Read the model definition and answer for the solid it produces. Units are mm, in the model's axes. Give positions to 0.01 mm unless a question says otherwise; leave off trailing zeros. Write each loop counter-clockwise with the first axis right and the second up, starting at its lowest first coordinate (ties: lowest second). Pieces come first, ordered by that corner, then holes. Notation, with made-up numbers: (52, 12) -> (69, 12) arc R30 ccw to (69, 50) -> close; hole circle Ø7 at (0.25, 11.25). An arc over 180 degrees is marked (long way). Use a Markdown table: item, result.
from build123d import *

# Parameters (mm, degrees)
F0_R     = 10.25
F0_R_2   = 11.173899
F1_DEPTH = 40


with BuildPart() as f1:
    # F0 (on Top) → F1 (new body)
    with BuildSketch(Plane.XY):
        with BuildLine():
            Line((-240, -166), (240, -166))
            ThreePointArc((240, -166), (247.071068, -163.071068), (250, -156))
            Line((250, -156), (250, 156))
            ThreePointArc((250, 156), (247.071068, 163.071068), (240, 166))
            Line((240, 166), (-240, 166))
            ThreePointArc((-240, 166), (-247.071068, 163.071068), (-250, 156))
            Line((-250, 156), (-250, -156))
            ThreePointArc((-250, -156), (-247.071068, -163.071068), (-240, -166))
        make_face()
        with Locations((-215, -120)):
            Circle(F0_R, mode=Mode.SUBTRACT)
        with Locations((-155, -120)):
            Circle(F0_R, mode=Mode.SUBTRACT)
        with Locations((-95, -120)):
            Circle(F0_R, mode=Mode.SUBTRACT)
        with Locations((-35, -120)):
            Circle(F0_R, mode=Mode.SUBTRACT)
        with Locations((-215, -60)):
            Circle(F0_R, mode=Mode.SUBTRACT)
        with Locations((-155, -60)):
            Circle(F0_R_2, mode=Mode.SUBTRACT)
        with Locations((-95, -60)):
            Circle(F0_R, mode=Mode.SUBTRACT)
        with Locations((-35, -60)):
            Circle(F0_R, mode=Mode.SUBTRACT)
        with Locations((25, -120)):
            Circle(F0_R, mode=Mode.SUBTRACT)
        with Locations((85, -120)):
            Circle(F0_R, mode=Mode.SUBTRACT)
        with Locations((145, -120)):
            Circle(F0_R, mode=Mode.SUBTRACT)
        with Locations((205, -120)):
            Circle(F0_R, mode=Mode.SUBTRACT)
        with Locations((25, -60)):
            Circle(F0_R, mode=Mode.SUBTRACT)
        with Locations((85, -60)):
            Circle(F0_R, mode=Mode.SUBTRACT)
        with Locations((145, -60)):
            Circle(F0_R, mode=Mode.SUBTRACT)
        with Locations((205, -60)):
            Circle(F0_R, mode=Mode.SUBTRACT)
        with Locations((-215, 0)):
            Circle(F0_R, mode=Mode.SUBTRACT)
        with Locations((-155, 0)):
            Circle(F0_R, mode=Mode.SUBTRACT)
        with Locations((-215, 60)):
            Circle(F0_R, mode=Mode.SUBTRACT)
        with Locations((-155, 60)):
            Circle(F0_R, mode=Mode.SUBTRACT)
        with Locations((-95, 0)):
            Circle(F0_R, mode=Mode.SUBTRACT)
        with Locations((-35, 0)):
            Circle(F0_R, mode=Mode.SUBTRACT)
        with Locations((-95, 60)):
            Circle(F0_R, mode=Mode.SUBTRACT)
        with Locations((-35, 60)):
            Circle(F0_R, mode=Mode.SUBTRACT)
        with Locations((-215, 120)):
            Circle(F0_R, mode=Mode.SUBTRACT)
        with Locations((-155, 120)):
            Circle(F0_R, mode=Mode.SUBTRACT)
        with Locations((-95, 120)):
            Circle(F0_R, mode=Mode.SUBTRACT)
        with Locations((-35, 120)):
            Circle(F0_R, mode=Mode.SUBTRACT)
        with Locations((25, 0)):
            Circle(F0_R, mode=Mode.SUBTRACT)
        with Locations((85, 0)):
            Circle(F0_R, mode=Mode.SUBTRACT)
        with Locations((25, 60)):
            Circle(F0_R, mode=Mode.SUBTRACT)
        with Locations((85, 60)):
            Circle(F0_R, mode=Mode.SUBTRACT)
        with Locations((145, 0)):
            Circle(F0_R, mode=Mode.SUBTRACT)
        with Locations((205, 0)):
            Circle(F0_R, mode=Mode.SUBTRACT)
        with Locations((145, 60)):
            Circle(F0_R, mode=Mode.SUBTRACT)
        with Locations((205, 60)):
            Circle(F0_R, mode=Mode.SUBTRACT)
        with Locations((25, 120)):
            Circle(F0_R, mode=Mode.SUBTRACT)
        with Locations((85, 120)):
            Circle(F0_R, mode=Mode.SUBTRACT)
        with Locations((145, 120)):
            Circle(F0_R, mode=Mode.SUBTRACT)
        with Locations((205, 120)):
            Circle(F0_R, mode=Mode.SUBTRACT)
    extrude(amount=F1_DEPTH)


solid = f1.part
Item 1: This flat-tipped pin is pushed along its axis until it touches: P1, Ø18.5, axis at x = 205, y = -120, coming from the +Z side (3 decimals). Where does it stop, or does it pass through?
Return value:
| item | result |
|---|---|
| P1 | through |
Item 2: For a pull along Y with two mould halves and no side action, classify faces 1 (the face through (247.15, 162.99, 19.72)), 2 (the face through (-247.15, -162.99, 19.72)), 3 (the face through (-103.13, -66.24, 19.72)) as +Y half, -Y half, draft (parallel to the pull), parting line (faces both ways), or undercut.
Return value:
| item | result |
|---|---|
| face 1 | +Y half |
| face 2 | -Y half |
| face 3 | undercut |
Item 3: A cutting plane is placed at A-A (x = 85). Give the vertices of the cut face in (y, z), then the cut area to 3 significant figures.
Return value:
| item | result |
|---|---|
| outline | (-166, 0) -> (-130.25, 0) -> (-130.25, 40) -> (-166, 40) -> close; (-109.75, 0) -> (-70.25, 0) -> (-70.25, 40) -> (-109.75, 40) -> close; (-49.75, 0) -> (-10.25, 0) -> (-10.25, 40) -> (-49.75, 40) -> close; (10.25, 0) -> (49.75, 0) -> (49.75, 40) -> (10.25, 40) -> close; (70.25, 0) -> (109.75, 0) -> (109.75, 40) -> (70.25, 40) -> close; (130.25, 0) -> (166, 0) -> (166, 40) -> (130.25, 40) -> close |
| area | 9,180 mm^2 |
Item 4: A cutting plane is placed at C-C (x = -155). Give the vertices of the cut face in (y, z), then the cut area to 3 significant figures.
Return value:
| item | result |
|---|---|
| outline | (-166, 0) -> (-130.25, 0) -> (-130.25, 40) -> (-166, 40) -> close; (-109.75, 0) -> (-71.17, 0) -> (-71.17, 40) -> (-109.75, 40) -> close; (-48.83, 0) -> (-10.25, 0) -> (-10.25, 40) -> (-48.83, 40) -> close; (10.25, 0) -> (49.75, 0) -> (49.75, 40) -> (10.25, 40) -> close; (70.25, 0) -> (109.75, 0) -> (109.75, 40) -> (70.25, 40) -> close; (130.25, 0) -> (166, 0) -> (166, 40) -> (130.25, 40) -> close |
| area | 9,110 mm^2 |
Item 5: Straight lines are drawn through the part: line 1 along Y through (x, z) = (25, 14); line 2 along Y through (x, z) = (93, 29.5). For each, find the intervals that lie inside material, in ascending order. Write a range as [from, to].
Return value:
| item | result |
|---|---|
| line 1 | [-166, -130.25], [-109.75, -70.25], [-49.75, -10.25], [10.25, 49.75], [70.25, 109.75], [130.25, 166] |
| line 2 | [-166, -126.41], [-113.59, -66.41], [-53.59, -6.41], [6.41, 53.59], [66.41, 113.59], [126.41, 166] |
Item 6: A cutting plane is placed at B-B (y = -60). Count the separate pieces of the cut face and the enclosed holes in it, then the cut area to 3 significant figures.
Return value:
| item | result |
|---|---|
| separate pieces | 9 |
| enclosed holes | 0 |
| area | 13,400 mm^2 |
